```python
from build123d import *

# Parameters (mm, degrees)
BOSS_EXTRUDE1_DEPTH = 76.2
FILLET1_RADIUS      = 38.1
FILLET1_LENGTH      = 12.7
FILLET2_RADIUS      = 38.1
FILLET2_LENGTH      = 12.7


with BuildPart() as part:
    # Sketch2 → Boss-Extrude1 (new body)
    with BuildSketch(Plane(origin=(0, 0, 0), x_dir=(0, 0, -1), z_dir=(1, 0, 0))):
        with BuildLine():
            Line((-394.160701906, 0), (-306.172520882, 0))
            ThreePointArc((-306.172520882, 0), (-293.024513391, 1.730968025), (-280.772520882, 6.805909488))
            Line((-280.772520882, 6.805909488), (280.772520882, 331.014090512))
            ThreePointArc((280.772520882, 331.014090512), (293.024513391, 336.089031975), (306.172520882, 337.82))
            Line((306.172520882, 337.82), (470.360701906, 337.82))
            Line((470.360701906, 337.82), (470.360701906, 325.12))
            Line((470.360701906, 325.12), (306.172520882, 325.12))
            ThreePointArc((306.172520882, 325.12), (296.311515264, 323.821773982), (287.122520882, 320.015567884))
            Line((287.122520882, 320.015567884), (-274.422520882, -4.19261314))
            ThreePointArc((-274.422520882, -4.19261314), (-289.737511518, -10.536289969), (-306.172520882, -12.7))
            Line((-306.172520882, -12.7), (-394.160701906, -12.7))
            Line((-394.160701906, -12.7), (-394.160701906, 0))
        make_face()
    extrude(amount=BOSS_EXTRUDE1_DEPTH)

    # Fillet1: full round fillet: the end face becomes a half cylinder, R = half its width
    fillet1_face = Plane((38.1, -6.35, 394.160701906), x_dir=(0, -1, 0), z_dir=(0, 0, 1))  # on the end face: x along it, z out of the body
    fillet1_slab = fillet1_face.offset(-FILLET1_RADIUS / 2) * Box(FILLET1_LENGTH, 2 * FILLET1_RADIUS, FILLET1_RADIUS, mode=Mode.PRIVATE)  # the body's end, R deep
    fillet1_round = Plane((38.1, -6.35, 356.060701906), x_dir=(0, 0, 1), z_dir=(0, -1, 0)) * Cylinder(FILLET1_RADIUS, FILLET1_LENGTH, mode=Mode.PRIVATE)  # its axis R under the face
    add(fillet1_slab - fillet1_round, mode=Mode.SUBTRACT)

    # Fillet2: full round fillet: the end face becomes a half cylinder, R = half its width
    fillet2_face = Plane((38.1, 331.47, -470.360701906), x_dir=(0, 1, 0), z_dir=(0, 0, -1))  # on the end face: x along it, z out of the body
    fillet2_slab = fillet2_face.offset(-FILLET2_RADIUS / 2) * Box(FILLET2_LENGTH, 2 * FILLET2_RADIUS, FILLET2_RADIUS, mode=Mode.PRIVATE)  # the body's end, R deep
    fillet2_round = Plane((38.1, 331.47, -432.260701906), x_dir=(0, 0, -1), z_dir=(0, 1, 0)) * Cylinder(FILLET2_RADIUS, FILLET2_LENGTH, mode=Mode.PRIVATE)  # its axis R under the face
    add(fillet2_slab - fillet2_round, mode=Mode.SUBTRACT)

    # Sketch4 → 1 (1) Diameter Hole1 (revolve, cut)
    with BuildSketch(Plane(origin=(38.1, 0, 356.060701906), x_dir=(0, 0, 1), z_dir=(1, 0, 0))):
        Polygon((0, 0), (0, 12.7), (12.7, 12.7), (12.7, 0.635), (13.335, 0), align=None)
    revolve(axis=Axis((38.1, 6.35, 356.060701906), (0, -1, 0)), mode=Mode.SUBTRACT)

    # Sketch7 → 1 (1) Diameter Hole2 (revolve, cut)
    with BuildSketch(Plane(origin=(38.1, 325.12, -432.260701906), x_dir=(0, 0, -1), z_dir=(1, 0, 0))):
        Polygon((0, 0), (0, 12.7), (12.7, 12.7), (12.7, 0.635), (13.335, 0), align=None)
    revolve(axis=Axis((38.1, 318.77, -432.260701906), (0, 1, 0)), mode=Mode.SUBTRACT)


solid = part.part
```
Design review of the part built by this model. Coordinates are the model's own, in mm. A direction names the side the tool comes from. Coordinates: 2 decimals unless noted, no trailing zeros. Write each loop counter-clockwise with the first axis right and the second up, starting at its lowest first coordinate (ties: lowest second). Pieces come first, ordered by that corner, then holes. Notation, with made-up numbers: M 30.5,-1.75 L 50.5,-1.75 A5 cw 50.5,3.25 Z; hole C 64,80 d6. An arc over 180 degrees is marked long. Answer as a JSON object with one key per item and string values.
Item 1: Insertion check: pin 1 Ø4 at (x, y) = (57, 54) entering from +Z; pin 2 Ø23 at (x, z) = (22.5, 355) entering from +Y; pin 3 Ø1.5 at (x, y) = (48.5, 100) entering from +Z. Each pin has a flat end and moves straight along its axis. Give the tip position at first contact, or say it passes through.
Outcome:
{"pin 1": "z = 202.49", "pin 2": "y = 0", "pin 3": "z = 120.65"}
Item 2: Wall thickness on probe 1 along Z at (x, y) = (38.1, -5.25); probe 2 along Z at (x, y) = (38.1, -6.5); probe 3 along Y at (x, z) = (24.5, -330): over which ranges is each line inside the solid? List them lowest first.
Outcome:
{"probe 1": "276.33 to 343.36, 368.76 to 394.16", "probe 2": "278.81 to 343.36, 368.76 to 394.16", "probe 3": "325.12 to 337.82"}
Item 3: Draft analysis for pull direction Z (two halves, no side actions). For faces 3 (the flat face through (38, 0, 341)), 4 (the cylindrical face through (37.542, 331.703, -419.573)), 5 (the cylindrical face through (37.57, 323.86, -296.45)), 6 (the cylindrical face through (45.828, -6.583, 345.982)), state which applies: pulls with the +Z half, pulls with the -Z half, needs draft (parallel to the pull), parting line crosses it, or undercut.
Outcome:
{"face 3": "needs draft", "face 4": "undercut", "face 5": "pulls with the -Z half", "face 6": "undercut"}
Item 4: Add section A-A, the plane x = 38.1. Give the boundary of the cut face in (y, z) (3 decimals), and give its area (3 significant figures).
Outcome:
{"outline": "M -12.7,306.173 A63.5 ccw -4.193,274.423 L 320.016,-287.123 A38.1 cw 325.12,-306.173 L 325.12,-418.926 L 325.755,-419.561 L 337.82,-419.561 L 337.82,-306.173 A50.8 ccw 331.014,-280.773 L 6.806,280.773 A50.8 cw 0,306.173 L 0,342.726 L -0.635,343.361 L -12.7,343.361 Z; M -12.7,368.761 L -0.635,368.761 L 0,369.396 L 0,394.161 L -12.7,394.161 Z; M 325.12,-470.361 L 337.82,-470.361 L 337.82,-444.961 L 325.755,-444.961 L 325.12,-445.596 Z", "area": "11,500 mm²"}
Item 5: Add section B-B, the plane y = 28.5. Give the boundary of the cut face in (x, z), and give its area (3 significant figures).
Outcome:
{"outline": "M 0,217.8 L 76.2,217.8 L 76.2,243.2 L 0,243.2 Z", "area": "1,940 mm²"}
Item 6: Machinability: for faces 1 (the flat face through (38, 325.12, -389)), 2 (the cylindrical face through (37.57, 336.04, -292.84)), which of the approach directions +Z, -Z, +X, -X, +Y, -Y give a long, thin tool a straight path to every point of the face, cutting with its end or side? Answer none if there is none.
Outcome:
{"face 1": "-Z, +X, -X, -Y", "face 2": "+Z, +X, -X, +Y"}
Item 7: Add section C-C, the plane z = -199.5. Give the boundary of the cut face in (x, y), and give its area (3 significant figures).
Outcome:
{"outline": "M 0,269.43 L 76.2,269.43 L 76.2,284.09 L 0,284.09 Z", "area": "1,120 mm²"}
